The model under review builds one solid part; all positions refer to its coordinate system, in mm. A direction names the side the tool comes from. Coordinates: 2 decimals unless noted, no trailing zeros. Write each loop counter-clockwise with the first axis right and the second up, starting at its lowest first coordinate (ties: lowest second). Pieces come first, ordered by that corner, then holes. Notation, with made-up numbers: M -6,46 L 47,46 A17 ccw 47,77 Z; hole C 15.25,19 d7. An arc over 180 degrees is marked long. Answer as a JSON object with one key per item and string values.
Autodesk Inventor part; units mm, degrees
ref_plane "YZ Plane" through (0, 0, 0) normal (1, 0, 0) x (0, 1, 0)
ref_plane "XZ Plane" through (0, 0, 0) normal (0, 1, 0) x (-1, 0, 0)
ref_plane "XY Plane" through (0, 0, 0) normal (0, 0, 1) x (1, 0, 0)
sketch "スケッチ1" plane through (0, 0, 0) normal (0, 0, 1) x (1, 0, 0)
  line L0 (16, 16) -> (-16, 16)
  line L1 (-16, 16) -> (-16, -16)
  line L2 (-16, -16) -> (16, -16)
  line L3 (16, -16) -> (16, 16)
  line L4 (14.4, 14.4) -> (-14.4, 14.4)
  line L5 (-14.4, 14.4) -> (-14.4, -14.4)
  line L6 (-14.4, -14.4) -> (14.4, -14.4)
  line L7 (14.4, -14.4) -> (14.4, 14.4)
  point P0 (0, 0)
  dimension "d6" = 32
  dimension "d7" = 32
  dimension "d8" = 1.6
  dimension "d24" = 16
  dimension "d26" = 16
extrude "押し出し3" add sketch "スケッチ1" along normal blind 330
sketch "スケッチ7" plane through (16, -16, 0) normal (1, 0, 0) x (0, 0, -1)
  line L0 (0, 0) -> (0, 32)
  line L1 (0, 0) -> (-330, 0)
  point P0 (0, 16)
  point P1 (-189, 16)
  dimension "d15" = 189
  dimension "d16" = 16
hole "穴1" at (16, 0, 189) direction (-1, 0, 0) diameter 10.5 end through all
chamfer "面取り2" distance 32 angle 45 1 edges at (-16, 0, 330)
(1) Add section D-D on z = 53. Give the boundary of the cut face in (x, y), and give its area (3 significant figures).
Results list:
{"outline": "M -16,-16 L 16,-16 L 16,16 L -16,16 Z; hole M -14.4,-14.4 L 14.4,-14.4 L 14.4,14.4 L -14.4,14.4 Z", "area": "195 mm²"}
(2) Draft analysis for pull direction Y (two halves, no side actions). For faces 3 (the face through (0, 16, 163)), 4 (the face through (-15.2, -1.6, 184)), 5 (the face through (-16, 0, 147)), state which applies: released by +Y, released by -Y, zero draft, split by the parting line, or undercut.
Results list:
{"face 3": "released by +Y", "face 4": "undercut", "face 5": "zero draft"}
(3) For faces 1 (the face through (16, 0, 163)), 2 (the face through (0, 14.4, 162)), list the 3-axis set-ups (+Z, -Z, +X, -X, +Y, -Y) from which the entire face can be reached by the end or side of a thin tool; tool diameter is ignored.
Results list:
{"face 1": "+Z, -Z, +X, +Y, -Y", "face 2": "+Z, -Z"}
(4) Wall thickness on line 1 along X through (y, z) = (-9.5, 261.5); line 2 along Y through (x, z) = (15.3, 189): over which ranges is each line inside the solid? List them lowest first. Write a range as from..to.
Results list:
{"line 1": "-16..-14.4, 14.4..16", "line 2": "-16..-5.25, 5.25..16"}
(5) Add section B-B on y = -10. Give the boundary of the cut face in (x, z).
Results list:
{"outline": "M -16,0 L -14.4,0 L -14.4,299.6 L -16,298 Z; M 14.4,0 L 16,0 L 16,330 L 14.4,328.4 Z"}
(6) Add section C-C on z = 189. Give the boundary of the cut face in (x, y).
Results list:
{"outline": "M -16,-16 L 16,-16 L 16,-5.25 L 14.4,-5.25 L 14.4,-14.4 L -14.4,-14.4 L -14.4,-5.25 L -16,-5.25 Z; M -16,5.25 L -14.4,5.25 L -14.4,14.4 L 14.4,14.4 L 14.4,5.25 L 16,5.25 L 16,16 L -16,16 Z"}
(7) Add section A-A on x = -5.5. Give the boundary of the cut face in (y, z).
Results list:
{"outline": "M -16,0 L -14.4,0 L -14.4,308.5 L -16,308.5 Z; M 14.4,0 L 16,0 L 16,308.5 L 14.4,308.5 Z"}
(8) For pin 1 Ø3 at (x, y) = (11.5, 5) entering from -Z; pin 2 Ø13.5 at (y, z) = (0, 189) entering from -X, all flat-tipped, find the tip position at first contact; note any pin that passes through.
Results list:
{"pin 1": "through", "pin 2": "x = -16"}
